For this review, take the finished solid that the model builds, in its own axes (mm). Face numbers are marked on the shaded views. A direction names the side the tool comes from. Give positions to 0.01 mm unless a question says otherwise; leave off trailing zeros. Write each loop counter-clockwise with the first axis right and the second up, starting at its lowest first coordinate (ties: lowest second). Pieces come first, ordered by that corner, then holes. Notation, with made-up numbers: M -36,24.25 L -20,24.25 A19 cw -20,36.25 Z; hole C 50,85 d3. An arc over 180 degrees is marked long. One line per item, written item: value. Start each with the question number.
Item 1: Mouldability with a two-part tool opening along X and no side actions: class the marked faces 1, 2, 3 and 4 as released by +X, released by -X, zero draft, split by the parting line, or undercut.
Item 2: Clearance check with flat-ended pins moving along their axes: pin 1 Ø1 at (x, z) = (-8, 3) entering from -Y; pin 2 Ø5 at (y, z) = (-5, 8) entering from -X; pin 3 Ø3 at (x, z) = (6, 8) entering from -Y. State where each tip first meets the part, or that it passes through.
Item 3: Consider section C-C, the plane x = -8.5. Write out the cut boundary in (y, z) (3 decimals).
Item 4: Consider section D-D, the plane y = -6. Write out the cut boundary in (x, z) (3 decimals).
Item 5: Tool access review of the marked faces 5 and 6: name each direction out of +Z, -Z, +X, -X, +Y, -Y from which nothing blocks a thin tool from reaching the whole face with its end or side.
Item 6: To check wall thickness, follow probe 1 along X at (y, z) = (0, 3.25); probe 2 along X at (y, z) = (14.5, 8.5); probe 3 along Y at (x, z) = (-2.5, 3). State the ranges of each line that lie inside material, in increasing order.
Item 7: Consider section A-A, the plane x = -3.5. Write out the cut boundary in (y, z) (3 decimals).
Autodesk Inventor part; units mm, degrees
ref_plane "YZ Plane" through (0, 0, 0) normal (1, 0, 0) x (0, 1, 0)
ref_plane "XZ Plane" through (0, 0, 0) normal (0, 1, 0) x (-1, 0, 0)
ref_plane "XY Plane" through (0, 0, 0) normal (0, 0, 1) x (1, 0, 0)
sketch "Sketch1" plane through (0, 0, 0) normal (1, 0, 0) x (0, 1, 0)
  circle A0 centre (0, 0) radius 9.525
  circle A1 centre (0, 0) radius 28.575
  circle A2 centre (0, 0) radius 4.7625
  circle A3 centre (15.875, 41.275) radius 4.7625
  line L0 (15.875, 41.275) -> (27.6665, 7.4435)
  line L1 (-19.9525, 92.075) -> (-19.9525, 41.275)
  circle A4 centre (15.875, 41.275) radius 35.8275
  line L2 (15.875, 41.275) -> (6.87, 6.5977)
  line L3 (0, 0) -> (0, 75.4256) construction
  line L4 (15.875, 41.275) -> (-18.4298, 139.7)
  line L5 (-26.3025, 92.075) -> (-26.3025, 41.275)
  line L6 (-26.3025, 41.275) -> (-13.6025, 41.275)
  line L7 (-13.6025, 41.275) -> (-13.6025, 92.075)
  line L8 (-13.6025, 92.075) -> (-26.3025, 92.075)
  line L9 (-26.3025, 92.075) -> (-13.6025, 41.275) construction
  line L10 (-26.3025, 41.275) -> (-13.6025, 92.075) construction
  point P0 (-19.9525, 66.675)
  dimension "d0" = 19.05
  dimension "d1" = 19.05
  dimension "d2" = 9.525
  dimension "d3" = 9.525
  dimension "d4" = 15.875
  dimension "d5" = 41.275
  dimension "d6" = 33.772
  dimension "d7" = 50.8
  dimension "d8" = 139.7
  dimension "d9" = 12.7
sketch "Sketch4" plane through (0, 0, 0) normal (0, 0, 1) x (1, 0, 0)
  circle A0 centre (0, 0) radius 9.525
  circle A1 centre (0, 0) radius 4.7625
  circle A2 centre (0, 0) radius 28.575 construction
  line L0 (0, 0) -> (0, 28.575)
  line L1 (0, 0) -> (28.575, 0) construction
  line L2 (0, 0) -> (-28.575, 0) construction
  line L3 (0, 0) -> (0, -28.575) construction
  circle A3 centre (0, 0) radius 19.05 construction
  circle A4 centre (0, 0) radius 23.114 construction
  circle A5 centre (0, 0) radius 25.908 construction
  arc A6 (19.05, 0) -> (0, 9.525) centre (5.9807, -2.3261) ccw
  arc A7 (0, -23.114) -> (19.05, 0) centre (-0.3155, -3.4467) ccw
  arc A8 (-25.908, 0) -> (0, -23.114) centre (-0.411, 2.5022) ccw
  arc A9 (0, 28.575) -> (-25.908, 0) centre (0, 2.5425) ccw
  line L4 (0, 0) -> (9.525, 16.4978) construction
  line L5 (0, 0) -> (19.05, 0) construction
  line L6 (0, 9.525) -> (6.3187, 10.9443)
  dimension "d61" = 19.05
  dimension "d65" = 46.228
  dimension "d66" = 51.816
  dimension "d62" = 9.525
  dimension "d63" = 19.05
  dimension "d64" = 38.1
  dimension "d68" = 30
extrude "Extrusion3" add sketch "Sketch4" along normal blind 9.525 contours A0 | L6 A6 A7 A8 A9 L0
fillet "Fillet1" radius 6.35 1 edges at (6.3187, 10.9443, 4.7625)
fillet "Fillet2" radius 2.3813 1 edges at (0, 9.525, 4.7625)
sketch "Sketch5" plane through (0, 0, 0) normal (0, 0, -1) x (-1, 0, 0)
  line L0 (0, 12.5005) -> (0, 28.575)
  circle A0 centre (0, 0) radius 28.575
  dimension "d73" = 57.15
properties part number "Snail Cam"
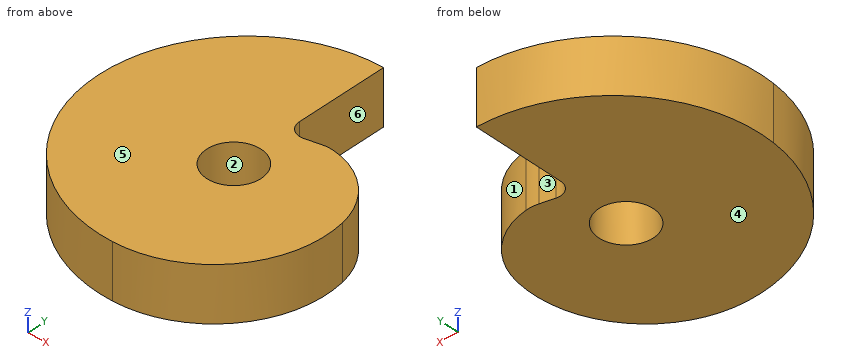
Model answer:
1. face 1: released by +X
1. face 2: undercut
1. face 3: undercut
1. face 4: zero draft
2. pin 1: stops at y = -22.12
2. pin 2: stops at x = -25.54
2. pin 3: stops at y = -22.52
3. outline: M -21.807,0 L 27.148,0 L 27.148,9.525 L -21.807,9.525 Z
4. outline: M -24.579,0 L 19.188,0 L 19.188,9.525 L -24.579,9.525 Z
5. face 5: +Z, +X, -X, +Y, -Y
5. face 6: +Z, -Z, +X, +Y
6. probe 1: x = -25.91 to -4.76, 4.76 to 19.05
6. probe 2: x = -23.12 to 0
6. probe 3: y = -23.03 to -4.05, 4.05 to 28.45
7. outline: M -22.93,0 L -3.23,0 L -3.23,9.525 L -22.93,9.525 Z; M 3.23,0 L 28.339,0 L 28.339,9.525 L 3.23,9.525 Z
